For this review, use the dimensioned drawing (mm, ordinates from the lowest corner) and the shaded views. Give positions to 0.01 mm unless a question says otherwise; leave off trailing zeros. Loops run counter-clockwise (first coordinate to the right, second up) from the corner with the lowest first, then second, coordinate; pieces in that order, holes last. Notation, with made-up numbers: (59.5, -30) -> (110.5, -30) arc R24 ccw to (110.5, -3) -> close; hole circle Ø11 at (-28.75, -24). An arc over 180 degrees is marked (long way). Write each question's results on one line, items separated by ' | '. Start each with the question number.
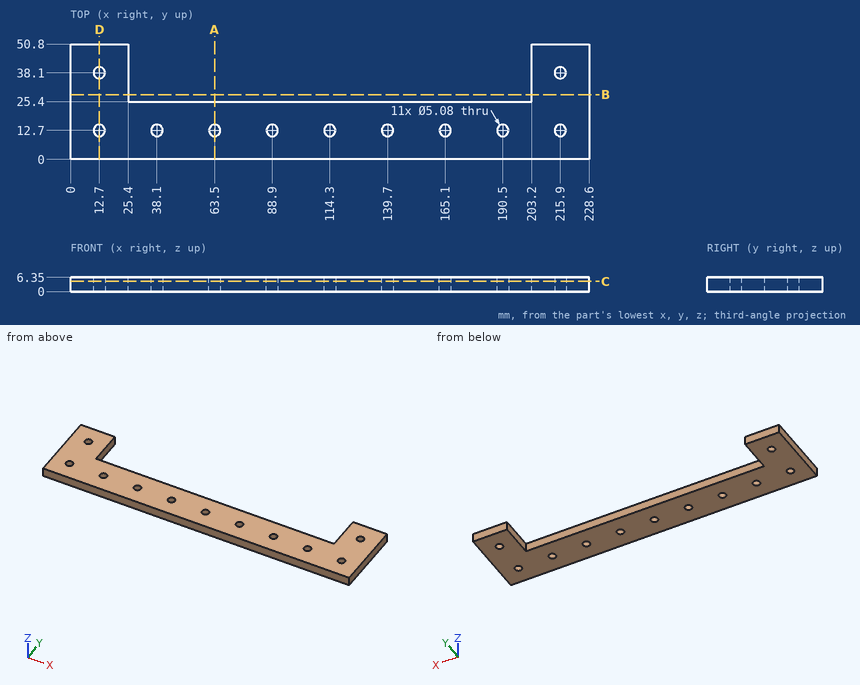
1. For pin 1 Ø1 at (x, y) = (113, 26.5) entering from -Z, flat-tipped, find the tip position at first contact; note if it passes through.
2. We need section A-A (x = 63.5). Write out the cut boundary in (y, z).
3. We need section C-C (z = 4.5). Count the separate pieces of the cut face and the enclosed holes in it, plus the area to 3 significant figures.
4. We need section D-D (x = 12.7). Write out the cut boundary in (y, z).
5. Wall thickness on L1, parallel to X at y = 28.5, z = 2.75; L2, parallel to X at y = 36, z = 4.5; L3, parallel to Y at x = 88.9, z = 1.5: over which ranges is each line inside the solid? List them lowest first.
6. We need section B-B (y = 28.5). Write out the cut boundary in (x, z).
Response:
1) pin 1: passes through
2) outline: (0, 0) -> (10.16, 0) -> (10.16, 6.35) -> (0, 6.35) -> close; (15.24, 0) -> (25.4, 0) -> (25.4, 6.35) -> (15.24, 6.35) -> close
3) separate pieces: 1 | enclosed holes: 11 | area: 6,870 mm2
4) outline: (0, 0) -> (10.16, 0) -> (10.16, 6.35) -> (0, 6.35) -> close; (15.24, 0) -> (35.56, 0) -> (35.56, 6.35) -> (15.24, 6.35) -> close; (40.64, 0) -> (50.8, 0) -> (50.8, 6.35) -> (40.64, 6.35) -> close
5) L1: x = 0 to 25.4, 203.2 to 228.6 | L2: x = 0 to 11.27, 14.13 to 25.4, 203.2 to 214.47, 217.33 to 228.6 | L3: y = 0 to 10.16, 15.24 to 25.4
6) outline: (0, 0) -> (25.4, 0) -> (25.4, 6.35) -> (0, 6.35) -> close; (203.2, 0) -> (228.6, 0) -> (228.6, 6.35) -> (203.2, 6.35) -> close
